The listing builds one solid part. Answer for the finished solid, in the listing's coordinates (mm). A direction names the side the tool comes from. Coordinates: 2 decimals unless noted, no trailing zeros. Order: outer loops, then holes, each group sorted by start corner. A loop starts at its lowest first (then second) coordinate and runs counter-clockwise, first axis right, second up. Notation, with made-up numbers: (56, 50) -> (108, 50) arc R33 ccw to (108, 88) -> close; hole circle Ø10 at (87, 8). An arc over 180 degrees is marked (long way). Return JSON: item names as keys, results as strings.
from build123d import *

# Parameters (mm, degrees)
SKETCH1_W           = 66.3
SKETCH1_H           = 110
BOSS_EXTRUDE1_DEPTH = 1.25
SKETCH2_W           = 2.5
SKETCH2_H           = 2.5
BOSS_EXTRUDE2_DEPTH = 5
SKETCH3_W           = 56.3
SKETCH3_H           = 100
CUT_EXTRUDE1_DEPTH  = 0.6


with BuildPart() as part:
    # Sketch1 → Boss-Extrude1 (new body)
    with BuildSketch(Plane.XY):
        with Locations((33.15, 55)):
            Rectangle(SKETCH1_W, SKETCH1_H)
    extrude(amount=BOSS_EXTRUDE1_DEPTH)

    # Sketch2 → Boss-Extrude2 (add)
    with BuildSketch(Plane.XY.offset(1.25)):
        with Locations((9.8, 2.5)):
            Rectangle(SKETCH2_W, SKETCH2_H)
        with Locations((9.8, 107.5)):
            Rectangle(SKETCH2_W, SKETCH2_H)
        with Locations((63.8, 55)):
            Rectangle(SKETCH2_W, SKETCH2_H)
    extrude(amount=BOSS_EXTRUDE2_DEPTH)

    # Sketch3 → Cut-Extrude1 (cut)
    with BuildSketch(Plane.XY.offset(1.25)):
        with Locations((33.15, 55)):
            Rectangle(SKETCH3_W, SKETCH3_H)
    extrude(amount=-CUT_EXTRUDE1_DEPTH, mode=Mode.SUBTRACT)


solid = part.part
1. The part is cut by section C-C on x = 60. Give the vertices of the cut face in (y, z).
Answer block:
{"outline": "(0, 0) -> (110, 0) -> (110, 1.25) -> (105, 1.25) -> (105, 0.65) -> (5, 0.65) -> (5, 1.25) -> (0, 1.25) -> close"}
2. The part is cut by section B-B on z = 2.25. Give the vertices of the cut face in (x, y), and give its area (4 significant figures).
Answer block:
{"outline": "(8.55, 1.25) -> (11.05, 1.25) -> (11.05, 3.75) -> (8.55, 3.75) -> close; (8.55, 106.25) -> (11.05, 106.25) -> (11.05, 108.75) -> (8.55, 108.75) -> close; (62.55, 53.75) -> (65.05, 53.75) -> (65.05, 56.25) -> (62.55, 56.25) -> close", "area": "18.75 mm2"}
3. Each of these flat-tipped pins is pushed along its axis until it touches: pin 1 Ø2 at (x, z) = (9.5, 4.5) entering from +Y; pin 2 Ø2 at (x, y) = (43.5, 68.5) entering from +Z; pin 3 Ø1 at (y, z) = (46, 2) entering from +X; pin 4 Ø2 at (y, z) = (55.5, 3.5) entering from +X. Where does it stop, or does it pass through?
Answer block:
{"pin 1": "stops at y = 108.75", "pin 2": "stops at z = 0.65", "pin 3": "passes through", "pin 4": "stops at x = 65.05"}
4. The part is cut by section A-A on y = 25. Give the vertices of the cut face in (x, z).
Answer block:
{"outline": "(0, 0) -> (66.3, 0) -> (66.3, 1.25) -> (61.3, 1.25) -> (61.3, 0.65) -> (5, 0.65) -> (5, 1.25) -> (0, 1.25) -> close"}
5. For faces 1 (the face through (10, 106.25, 4)), 2 (the face through (62.55, 55, 4)), 3 (the face through (64, 56.25, 4)), 4 (the face through (65.05, 55, 4)), 5 (the face through (10, 1.25, 4)), determine the directions among +Z, -Z, +X, -X, +Y, -Y from which every point of the face is accessible in a straight line to the end or side of a thin tool.
Answer block:
{"face 1": "+Z, +X, -X", "face 2": "+Z, -X, +Y, -Y", "face 3": "+Z, +X, -X, +Y", "face 4": "+Z, +X, +Y, -Y", "face 5": "+Z, +X, -X, -Y"}
6. Consider line 1 (Y direction, x = 7, z = 1); line 2 (Y direction, x = 11, z = 4.5); line 3 (X direction, y = 24.5, z = 0.75). Determine where each line is inside the solid, lowest interval first. Write a range as from..to.
Answer block:
{"line 1": "y = 0..5, 105..110", "line 2": "y = 1.25..3.75, 106.25..108.75", "line 3": "x = 0..5, 61.3..66.3"}
